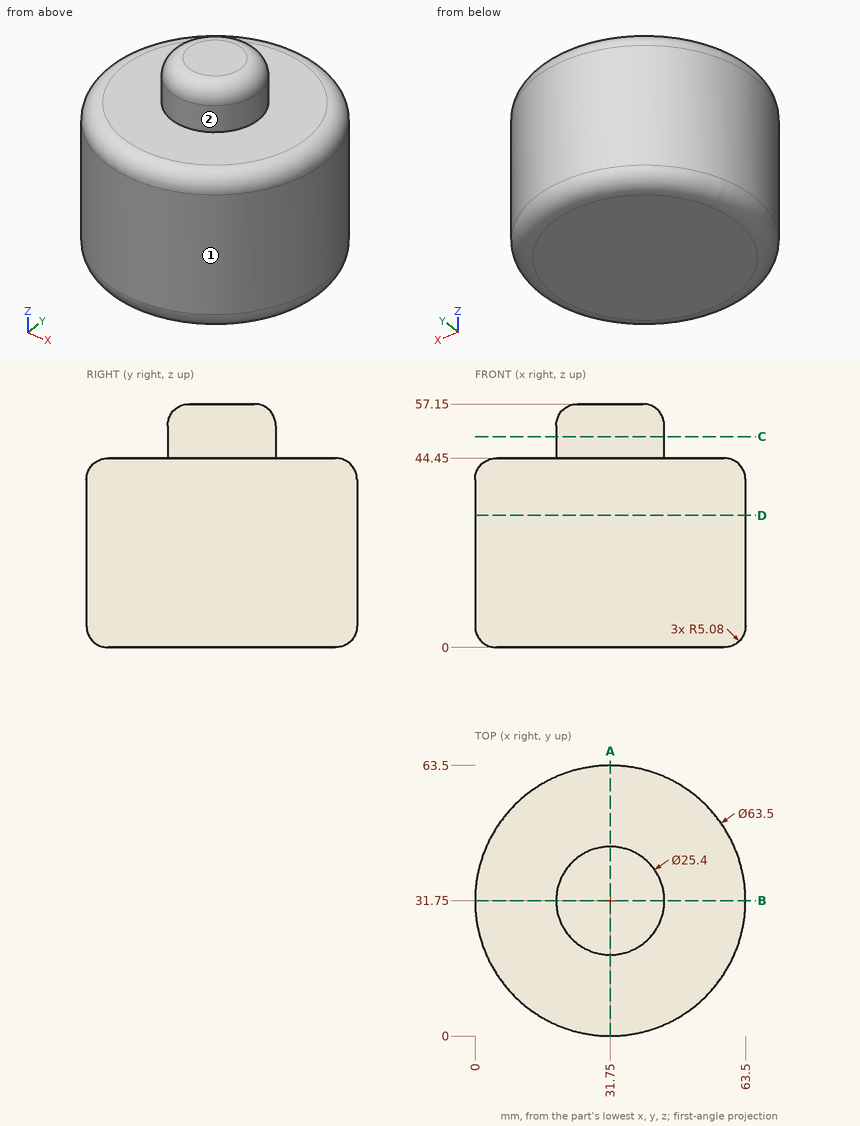
Drawing for the job (mm, zero at the part's lowest x, y, z). A direction names the side the tool comes from. Round coordinates to 2 decimals unless told otherwise and drop trailing zeros. Loops run counter-clockwise (first coordinate to the right, second up) from the corner with the lowest first, then second, coordinate; pieces in that order, holes last.
1. Wall check: probe 1 along Z at (x, y) = (30.5, 13); probe 2 along Y at (x, z) = (32.5, 15); probe 3 along Z at (x, y) = (22.5, 60). Give the ranges that are in metal, low to high.
Check values:
probe 1: z = 0 to 44.45
probe 2: y = 0.01 to 63.49
probe 3: z = 1.02 to 43.43
2. Band-saw the part on C-C, the plane z = 49.5. List the corners of the cut face in (x, y).
Check values:
outline: circle Ø25.4 at (31.75, 31.75)
3. Band-saw the part on D-D, the plane z = 31. List the corners of the cut face in (x, y).
Check values:
outline: circle Ø63.5 at (31.75, 31.75)
4. Tool access for the marked faces 1 and 2: list every direction of +Z, -Z, +X, -X, +Y, -Y with a clear straight run to the whole face (end or side of a thin tool).
Check values:
face 1: +Z, -Z
face 2: +Z
5. Band-saw the part on A-A, the plane x = 31.75. List the corners of the cut face in (y, z), and give its area (3 significant figures).
Check values:
outline: (0, 5.08) arc R5.08 ccw to (5.08, 0) - (58.42, 0) arc R5.08 ccw to (63.5, 5.08) - (63.5, 39.37) arc R5.08 ccw to (58.42, 44.45) - (44.45, 44.45) - (44.45, 52.07) arc R5.08 ccw to (39.37, 57.15) - (24.13, 57.15) arc R5.08 ccw to (19.05, 52.07) - (19.05, 44.45) - (5.08, 44.45) arc R5.08 ccw to (0, 39.37) - close
area: 3,110 mm2
6. Drop flat-ended pins along their axis: P1, Ø8, axis at y = 47, z = 49.5, coming from the -X side; P2, Ø5, axis at y = 41, z = 39, coming from the -X side; P3, Ø1.5, axis at x = 36.5, z = 21.5, coming from the -Y side; P4, Ø10, axis at x = 21.5, y = 24.5, coming from the +Z side. Give the stop position or say it passes through.
Check values:
P1: stops at x = 25.86
P2: stops at x = 0.73
P3: stops at y = 0.25
P4: stops at z = 57.15
